Here's how the part is built. I have some questions about the finished solid (model axes, mm). Round coordinates to 2 decimals unless told otherwise and drop trailing zeros. Write each loop counter-clockwise with the first axis right and the second up, starting at its lowest first coordinate (ties: lowest second). Pieces come first, ordered by that corner, then holes. Notation, with made-up numbers: (28.25, 64) - (66.25, 64) arc R16 ccw to (66.25, 86) - close; hole circle Ø3 at (4, 51). An arc over 180 degrees is marked (long way). Write item = value, one per line. Start each with the question number.
Item 1: If we section it at C-C (z = -80): Please give me the cut outline in (x, y).
Item 2: For P1, Ø12, axis at x = 42, y = -9, coming from the -Z side; P2, Ø5.5, axis at x = -55.5, z = 67.5, coming from the +Y side; P3, Ø1.5, axis at y = -4.5, z = 67, coming from the -X side, each with a flat end and sliding along its axis, tell me the tip position at first contact or that it passes through.
Item 3: If we section it at B-B (x = 0): Please give me the cut outline in (y, z).
Item 4: If we section it at D-D (x = -98.5): Please give me the cut outline in (y, z), and give its area (3 significant figures).
Item 5: If we section it at A-A (y = -11.25): Please give me the cut outline in (x, z) (3 decimals).
Item 6: If I drill on line 1 along Z through (x, y) = (130, -8); line 2 along X through (y, z) = (1.25, -76.5); line 3 along Y through (x, z) = (0, 165), over which ranges is the centre line in solid material (lowest first)? Write a range as [from, to].
```python
from build123d import *

# Parameters (mm, degrees)
BOSS_EXTRUDE1_DEPTH      = 335.28
BOSS_EXTRUDE1_DEPTH_BACK = 335.28
SKETCH1_R                = 7
SKETCH1_R_2              = 6
SKETCH3_W                = 298.43
SKETCH3_H                = 5
BOSS_EXTRUDE2_DEPTH      = 10
BOSS_EXTRUDE3_START      = -70.13
BOSS_EXTRUDE3_DEPTH      = 5


with BuildPart() as part:
    # Sketch1 → Boss-Extrude1 (new, two sides: drawn at the far end of the back side and taken through both)
    with BuildSketch(Plane.XY.offset(-BOSS_EXTRUDE1_DEPTH_BACK)):
        Circle(SKETCH1_R)
        Circle(SKETCH1_R_2, mode=Mode.SUBTRACT)
    extrude(amount=BOSS_EXTRUDE1_DEPTH + BOSS_EXTRUDE1_DEPTH_BACK)



with BuildPart() as body_2:
    # Sketch3 → Boss-Extrude2 (new body)
    with BuildSketch(Plane(origin=(0, -7, 0), x_dir=(1, 0, 0), z_dir=(0, 1, 0))):
        with Locations((0, 67.63)):
            Rectangle(SKETCH3_W, SKETCH3_H)
    boss_extrude2 = extrude(amount=-BOSS_EXTRUDE2_DEPTH)


with BuildPart() as part_1:
    add(part.part)

    add(body_2.part)  # Boss-Extrude3 merges body 2
    # Boss-Extrude3: read off the stored shape, not the designer's step
    # Boss-Extrude3 outline → Boss-Extrude3 (add)
    with BuildSketch(Plane.XY.offset(BOSS_EXTRUDE3_START)):
        with BuildLine():
            Line((7, -7), (7, 0))
            ThreePointArc((7, 0), (4.94974746, -4.949747477), (-2.4e-08, -7))
            Line((-2.4e-08, -7), (7, -7))
        make_face()
        with BuildLine():
            ThreePointArc((-2.4e-08, -7), (-4.949747477, -4.94974746), (-7, 0))
            Line((-7, 0), (-7, -7))
            Line((-7, -7), (-2.4e-08, -7))
        make_face()
    boss_extrude3 = extrude(amount=BOSS_EXTRUDE3_DEPTH)

    # Mirror12: Boss-Extrude2, Boss-Extrude3 across plane
    add(boss_extrude2.mirror(Plane.XY))
    add(boss_extrude3.mirror(Plane.XY))


solid = part_1.part
```
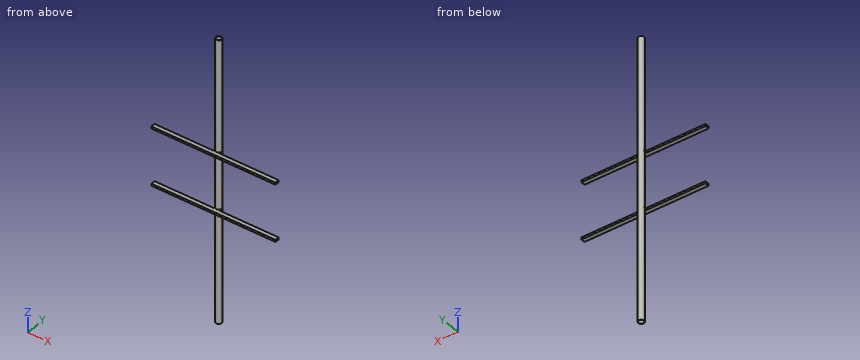
Reply:
q1.outline = circle Ø14 at (0, 0); hole circle Ø12 at (0, 0)
q2.P1 = -70.13
q2.P2 = -7
q2.P3 = -7
q3.outline = (-17, -70.13) - (-7, -70.13) - (-7, -335.28) - (-6, -335.28) - (-6, 335.28) - (-7, 335.28) - (-7, 70.13) - (-17, 70.13) - (-17, 65.13) - (-7, 65.13) - (-7, -65.13) - (-17, -65.13) - close; (6, -335.28) - (7, -335.28) - (7, 335.28) - (6, 335.28) - close
q4.outline = (-17, -70.13) - (-7, -70.13) - (-7, -65.13) - (-17, -65.13) - close; (-17, 65.13) - (-7, 65.13) - (-7, 70.13) - (-17, 70.13) - close
q4.area = 100 mm2
q5.outline = (-149.215, -70.13) - (149.215, -70.13) - (149.215, -65.13) - (-149.215, -65.13) - close; (-149.215, 65.13) - (149.215, 65.13) - (149.215, 70.13) - (-149.215, 70.13) - close
q6.line_1 = [-70.13, -65.13], [65.13, 70.13]
q6.line_2 = [-6.89, -5.87], [5.87, 6.89]
q6.line_3 = [-7, -6], [6, 7]
